Here's how the part is built. I have some questions about the finished solid (model axes, mm). Face numbers are marked on the shaded views. A direction names the side the tool comes from. Give positions to 0.01 mm unless a question says otherwise; leave off trailing zeros. Order: outer loops, then holes, each group sorted by start corner. A loop starts at its lowest first (then second) coordinate and runs counter-clockwise, first axis right, second up. Notation, with made-up numbers: (52.5, 36) - (76.5, 36) arc R18 ccw to (76.5, 60) - close; hole circle Ø9 at (65.25, -37.5). An arc over 180 degrees is marked (long way). One line per question, with ' | ' between items.
from build123d import *

# Parameters (mm, degrees)
SKIZZE1_R                       = 3.5
AUFSATZ_LINEAR_AUSTRAGEN1_DEPTH = 1
SKIZZE2_R                       = 1.45
AUFSATZ_LINEAR_AUSTRAGEN2_DEPTH = 20
SKIZZE3_W                       = 0.5
SKIZZE3_H                       = 3
SCHNITT_LINEAR_AUSTRAGEN1_DEPTH = 17
SKIZZE4_R                       = 0.5
SCHNITT_LINEAR_AUSTRAGEN2_DEPTH = 17


with BuildPart() as part:
    # Skizze1 → Aufsatz-Linear austragen1 (new body)
    with BuildSketch(Plane(origin=(0, 0, 0), x_dir=(1, 0, 0), z_dir=(0, 1, 0))):
        with Locations(Location((0, 0, 0), (0, 0, 270))):
            Circle(SKIZZE1_R)
    extrude(amount=AUFSATZ_LINEAR_AUSTRAGEN1_DEPTH)

    # Skizze2 → Aufsatz-Linear austragen2 (add)
    with BuildSketch(Plane(origin=(0, 1, 0), x_dir=(1, 0, 0), z_dir=(0, 1, 0))):
        with Locations(Location((0, 0, 0), (0, 0, 270))):
            Circle(SKIZZE2_R)
    extrude(amount=AUFSATZ_LINEAR_AUSTRAGEN2_DEPTH)

    # Skizze3 → Schnitt-Linear austragen1 (cut)
    with BuildSketch(Plane(origin=(0, 21, 0), x_dir=(1, 0, 0), z_dir=(0, 1, 0))):
        Rectangle(SKIZZE3_W, SKIZZE3_H)
    extrude(amount=-SCHNITT_LINEAR_AUSTRAGEN1_DEPTH, mode=Mode.SUBTRACT)

    # Skizze4 → Schnitt-Linear austragen2 (cut)
    with BuildSketch(Plane(origin=(0, 21, 0), x_dir=(1, 0, 0), z_dir=(0, 1, 0))):
        Circle(SKIZZE4_R)
    extrude(amount=-SCHNITT_LINEAR_AUSTRAGEN2_DEPTH, mode=Mode.SUBTRACT)


solid = part.part
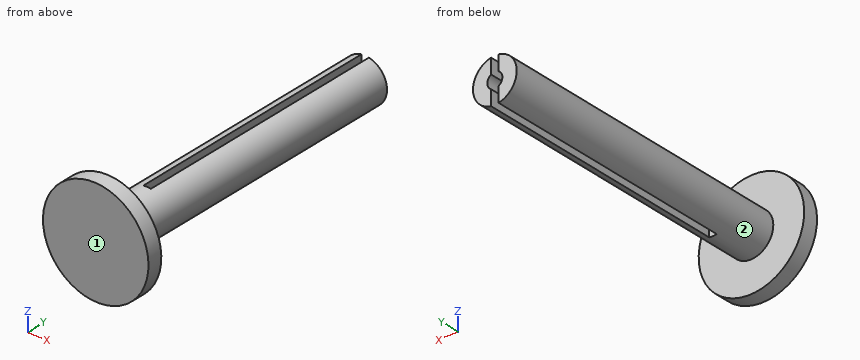
1) I want a section at C-C (x = 0). List the corners of the cut face in (y, z) for me.
Model answer:
outline: (0, -3.5) - (1, -3.5) - (1, -1.45) - (4, -1.45) - (4, 1.45) - (1, 1.45) - (1, 3.5) - (0, 3.5) - close
2) I'm going to push flat-ended pins straight in: P1, Ø4, axis at x = 1.5, y = 14, coming from the -Z side; P2, Ø0.8, axis at y = 10, z = -1, coming from the -X side; P3, Ø2, axis at x = 1, z = 1.5, coming from the +Y side; P4, Ø1, axis at x = -0.5, y = 2.5, coming from the +Z side. Where does each tip first touch, or does it pass through?
Model answer:
P1: stops at z = -1.43 | P2: stops at x = -1.32 | P3: stops at y = 21 | P4: stops at z = 1.45
3) Please list where these lines run through material, in increasing order: L1, parallel to Y at x = -2, z = 1.5; L2, parallel to X at y = 11.25, z = 1.25; L3, parallel to X at y = 8.5, z = 1.
Model answer:
L1: y = 0 to 1 | L2: x = -0.73 to -0.25, 0.25 to 0.73 | L3: x = -1.05 to -0.25, 0.25 to 1.05
4) I want a section at D-D (y = 2.75). List the corners of the cut face in (x, z) for me.
Model answer:
outline: circle Ø2.9 at (0, 0)
5) I want a section at A-A (y = 12). List the corners of the cut face in (x, z) for me.
Model answer:
outline: (-0.25, -1.43) - (-0.25, -0.43) arc R0.5 cw to (-0.25, 0.43) - (-0.25, 1.43) arc R1.45 ccw to start; (0.25, -1.43) arc R1.45 ccw to (0.25, 1.43) - (0.25, 0.43) arc R0.5 cw to (0.25, -0.43) - close
6) On a 3-axis mill with a long thin cutter (end or side, diameter ignored), from which of +Z, -Z, +X, -X, +Y, -Y can I reach the whole of each face in a straight line? I mean the marked faces 1 and 2. Say none if no direction works.
Model answer:
face 1: +Z, -Z, +X, -X, -Y | face 2: +Y
7) I want a section at B-B (z = 0). List the corners of the cut face in (x, y) for me.
Model answer:
outline: (-3.5, 0) - (3.5, 0) - (3.5, 1) - (1.45, 1) - (1.45, 21) - (0.5, 21) - (0.5, 4) - (-0.5, 4) - (-0.5, 21) - (-1.45, 21) - (-1.45, 1) - (-3.5, 1) - close
